Part model, mm, in its own coordinate system. A direction names the side the tool comes from. Coordinates: 2 decimals unless noted, no trailing zeros. Loops run counter-clockwise (first coordinate to the right, second up) from the corner with the lowest first, then second, coordinate; pieces in that order, holes last. Notation, with made-up numbers: M -14,4 L 23,4 A12 ccw 23,12 Z; hole C -1,23 d4. An arc over 180 degrees is marked long. Use a Markdown table: item, result. Add a question column.
1) Tool access for faces 1 (the flat face through (35, 7.747, 5)), 2 (the cylindrical face through (29.01, 10.03, 19.1)), 3 (the cylindrical face through (30.663, 9.883, 75.952)): list every direction of +Z, -Z, +X, -X, +Y, -Y with a clear straight run to the whole face (end or side of a thin tool).
2) Pull direction Z, two halves, no side cores. Call faces 4 (the cylindrical face through (29.01, -9.22, 60.68)), 5 (the cylindrical face through (35.188, -5.905, 14.539)), 6 (the cylindrical face through (30.663, -9.167, 75.952)), 7 (the flat face through (27.226, 6, 52)): released by +Z, released by -Z, zero draft, split by the parting line, or undercut.
3) Band-saw the part on B-B (x = 34.75). List the corners of the cut face in (y, z), plus the area to 3 significant figures.
4) Pin check, flat tips, straight feed: pin 1 Ø1.5 at (y, z) = (15, 60.5) entering from +X; pin 2 Ø4 at (y, z) = (-13, 12) entering from +X; pin 3 Ø4.5 at (y, z) = (1.5, 4.5) entering from +X. Stop position of each tip, or through.
5) Wall check: probe 1 along Z at (x, y) = (27.5, 5); probe 2 along Z at (x, y) = (28.5, -9); probe 3 along X at (y, z) = (-11.5, 35). Give the ranges that are in metal, low to high. Write a range as from..to.
6) Band-saw the part on C-C (y = 0). List the corners of the cut face in (x, z) (3 decimals), plus the area to 3 significant figures.
7) Band-saw the part on A-A (z = 7). List the corners of the cut face in (x, y) (3 decimals).
8) Band-saw the part on D-D (y = -4.5). List the corners of the cut face in (x, z).
Autodesk Inventor part; units mm, degrees
ref_plane "YZ Plane" through (0, 0, 0) normal (1, 0, 0) x (0, 1, 0)
ref_plane "XZ Plane" through (0, 0, 0) normal (0, 1, 0) x (-1, 0, 0)
ref_plane "XY Plane" through (0, 0, 0) normal (0, 0, 1) x (1, 0, 0)
sketch "Sketch1" plane through (0, 0, 0) normal (0, 0, 1) x (1, 0, 0)
  arc A0 (32.3009, 19.05) -> (32.3009, -19.05) centre (0, 0) ccw construction
  line L0 (0, 0) -> (25.8762, 0) construction
  line L1 (25.8762, 0) -> (25.8762, 19.05)
  line L2 (25.8762, 19.05) -> (32.3009, 19.05)
  line L3 (38.5763, 19.05) -> (38.5763, -19.05) construction
  line L4 (38.5763, -19.05) -> (32.3009, -19.05) construction
  line L5 (25.8762, -19.05) -> (25.8762, 0)
  line L6 (32.3009, 19.05) -> (38.5763, 19.05) construction
  line L7 (32.3009, -19.05) -> (25.8762, -19.05)
  arc A1 (32.3009, -19.05) -> (36.9585, -6.35) centre (0, 0) ccw
  line L8 (30.6388, 19.05) -> (30.6388, -19.05) construction
  line L9 (25.8762, 6.35) -> (36.9585, 6.35) construction
  line L10 (25.8762, -6.35) -> (36.9585, -6.35) construction
  arc A2 (36.9585, 6.35) -> (32.3009, 19.05) centre (0, 0) ccw
  arc A3 (36.9585, -6.35) -> (36.9585, 6.35) centre (0, 0) ccw
  line L11 (36.9585, 6.35) -> (36.9585, -6.35) construction
  point P0 (30.6388, 9.525)
  point P1 (30.6388, -9.525)
  dimension "d0" = 75
  dimension "d1" = 25.8762
  dimension "d2" = 19.05
  dimension "d3" = 19.05
  dimension "d4" = 12.7
  dimension "d5" = 4.7625
  dimension "d6" = 19.05
  dimension "d7" = 9.525
  dimension "d8" = 9.525
  dimension "d9" = 12.7
  dimension "d10" = 6.35
extrude "Extrusion1" add sketch "Sketch1" along normal blind 82.3912
hole "Hole1" at (30.6388, 9.525, 0) at (30.6388, -9.525, 0) direction (0, 0, 1) diameter 3.302 depth 9.525 tip angle 118
sketch "Sketch2" plane through (25.8762, -19.05, 0) normal (-1, 0, 0) x (0, 0, 1)
  line L0 (0, 38.1) -> (82.3912, 38.1)
  line L1 (0, 19.05) -> (9.525, 19.05) construction
  circle A0 centre (9.525, 19.05) radius 6
  line L2 (82.3912, 38.1) -> (82.3912, 0)
  line L3 (9.525, 19.05) -> (56.515, 19.05) construction
  circle A1 centre (56.515, 19.05) radius 8.5
  circle A2 centre (9.525, 19.05) radius 25.4
  circle A3 centre (56.515, 19.05) radius 21.59
  circle A4 centre (56.515, 19.05) radius 7.1437
  dimension "d20" = 9.525
  dimension "d21" = 12
  dimension "d24" = 17
  dimension "d52" = 50.8
  dimension "d53" = 43.18
  dimension "d55" = 14.2875
extrude "Extrusion2" cut sketch "Sketch2" against normal through all contours A0 | A4
sketch "Sketch3" plane through (0, 0, 0) normal (0, 0, -1) x (-1, 0, 0)
  line L0 (-25.8762, -19.05) -> (-25.8762, 19.05)
  arc A0 (-32.3009, 19.05) -> (-32.3009, -19.05) centre (0, 0) ccw
  line L1 (-25.8762, 0) -> (-37.5, 0)
  line L2 (-33.69, 0) -> (-33.69, 7.747)
  line L3 (-33.69, 7.747) -> (-36.6911, 7.747)
  line L4 (-33.69, 0) -> (-33.69, -7.747)
  line L5 (-33.69, -7.747) -> (-36.6911, -7.747)
  line L6 (-37.5, 5.6093) -> (-37.5, -5.6093) construction
  dimension "d28" = 3.81
  dimension "d29" = 15.494
extrude "Extrusion3" cut sketch "Sketch3" against normal blind 17.272
fillet "Fillet1" radius 7.747 2 edges at (35.1905, -7.747, 17.272) (35.1905, 7.747, 17.272)
sketch "Sketch4" plane through (0, 0, 82.3912) normal (0, 0, 1) x (1, 0, 0)
  line L0 (25.8762, 19.05) -> (25.8762, -19.05)
  line L1 (25.8762, -19.05) -> (32.3009, -19.05)
  arc A0 (32.3009, -19.05) -> (32.3009, 19.05) centre (0, 0) ccw
  line L2 (32.3009, 19.05) -> (25.8762, 19.05)
  line L3 (32.2263, 19.05) -> (32.2263, -19.05)
  dimension "d33" = 6.35
extrude "Extrusion4" cut sketch "Sketch4" against normal blind 65.2475 contours L2 A0 L1 L3
sketch "Sketch5" plane through (32.2263, -19.05, 82.3912) normal (1, 0, 0) x (0, 0, -1)
  line L0 (65.2475, 0) -> (0, 0)
  line L1 (65.2475, 0) -> (65.2475, 38.1)
  line L2 (0, 38.1) -> (65.2475, 38.1)
  line L3 (58.8975, 38.1) -> (58.8975, 0)
  line L4 (62.0725, 38.1) -> (62.0725, 0)
  line L5 (58.8975, 19.05) -> (65.2475, 19.05)
  point P0 (82.3912, 19.05)
  point P1 (62.0725, 28.575)
  point P2 (62.0725, 9.525)
  dimension "d36" = 6.35
  dimension "d37" = 19.05
  dimension "d38" = 9.525
hole "Hole2" at (32.2263, 9.525, 20.3187) at (32.2263, -9.525, 20.3187) direction (-1, 0, 0) diameter 2.6416 end through all
extrude "Extrusion6" cut sketch "Sketch2" against normal through all contours A1
extrude "Extrusion7" add sketch "Sketch2" against normal blind 1.35 contours A1
sketch "Sketch7" plane through (0, 0, 82.3912) normal (0, 0, 1) x (1, 0, 0)
  line L0 (32.2263, -19.05) -> (32.2263, 19.05)
  line L1 (25.8762, 19.05) -> (25.8762, -19.05)
  line L2 (29.0512, 19.05) -> (29.0513, -19.05) construction
  line L3 (25.8762, 0) -> (32.2263, 0) construction
  line L4 (32.2263, 19.05) -> (25.8762, 19.05)
  point P0 (0, 0)
  point P1 (29.0513, 9.525)
  point P2 (29.0513, -9.525)
  dimension "d60" = 9.525
hole "Hole3" at (29.0513, 9.525, 82.3912) at (29.0513, -9.525, 82.3912) direction (0, 0, -1) diameter 3.302 depth 12.7 tip angle 118
sketch "Sketch8" plane through (32.2263, -19.05, 82.3912) normal (1, 0, 0) x (0, 0, -1)
  circle A0 centre (25.8762, 19.05) radius 8.5
  line L0 (0, 38.1) -> (65.2475, 38.1)
  circle A1 centre (25.8763, 19.05) radius 11.3766 construction
  line L1 (25.8763, 19.05) -> (37.2528, 19.05) construction
  line L2 (25.8763, 19.05) -> (20.188, 28.9024) construction
  line L3 (25.8763, 19.05) -> (20.188, 9.1976) construction
  circle A2 centre (37.2528, 19.05) radius 3.9688 construction
  circle A3 centre (37.2528, 19.05) radius 2.0828 construction
  point P0 (82.3912, 19.05)
  point P1 (35.17, 19.05)
  point P2 (34.3763, 19.05)
  point P3 (33.2841, 19.05)
  dimension "d70" = 7.9375
  dimension "d71" = 4.1656
  dimension "d68" = 120
  dimension "d69" = 120
  dimension "d72" = 1.0922
  dimension "d73" = 0.7937
hole "Hole4" at (32.2263, 0, 45.1384) at (32.2263, -9.8524, 62.2033) at (32.2263, 9.8524, 62.2033) direction (-1, 0, 0) diameter 3.302 end through all
equation "\"d3\" = d2"
properties part number "Module Side Beam" material "Aluminum 6061"
Entries:
| question | item | result |
|---|---|---|
| 1 | face 1 | -Z, +X |
| 1 | face 2 | +X, -X |
| 1 | face 3 | +Z |
| 2 | face 4 | undercut |
| 2 | face 5 | released by -Z |
| 2 | face 6 | zero draft |
| 2 | face 7 | undercut |
| 3 | outline | M -14.1,0 L -7.75,0 L -7.75,9.53 A7.75 cw -1.4,17.14 L -14.1,17.14 Z; M 1.4,17.14 A7.75 cw 7.75,9.53 L 7.75,0 L 14.1,0 L 14.1,17.14 Z |
| 3 | area | 242 mm2 |
| 4 | pin 1 | x = 32.23 |
| 4 | pin 2 | x = 35.85 |
| 4 | pin 3 | x = 33.69 |
| 5 | probe 1 | 0..6.21, 12.84..49.64, 63.39..82.39 |
| 5 | probe 2 | 0..19.11, 21.53..60.79, 63.62..69.16 |
| 5 | probe 3 | 25.88..32.23 |
| 6 | outline | M 25.876,0 L 33.69,0 L 33.69,3.525 L 25.876,3.525 Z; M 25.876,15.525 L 33.69,15.525 L 33.69,17.144 L 32.226,17.144 L 32.226,43.487 L 25.876,43.487 Z; M 25.876,46.789 L 32.226,46.789 L 32.226,48.015 L 27.226,48.015 L 27.226,49.371 L 25.876,49.371 Z; M 25.876,63.659 L 27.226,63.659 L 27.226,65.015 L 32.226,65.015 L 32.226,82.391 L 25.876,82.391 Z |
| 6 | area | 329 mm2 |
| 7 | outline | M 25.876,-19.05 L 32.301,-19.05 A37.501 ccw 36.691,-7.747 L 33.69,-7.747 L 33.69,-5.443 L 25.876,-5.443 Z; M 25.876,5.443 L 33.69,5.443 L 33.69,7.747 L 36.691,7.747 A37.499 ccw 32.301,19.05 L 25.876,19.05 Z; hole C 30.639,-9.525 d3.302; hole C 30.639,9.525 d3.302 |
| 8 | outline | M 25.88,0 L 33.69,0 L 33.69,5.56 L 25.88,5.56 Z; M 25.88,13.49 L 33.69,13.49 L 33.69,15.83 L 37.23,15.83 L 37.23,17.14 L 32.23,17.14 L 32.23,49.3 L 27.23,49.3 L 27.23,50.97 L 25.88,50.97 Z; M 25.88,62.06 L 27.23,62.06 L 27.23,63.73 L 32.23,63.73 L 32.23,82.39 L 25.88,82.39 Z |
